The figure shows three views and two pictorial views of one solid part (mm, origin at its lowest corner). Answer the questions. A direction names the side the tool comes from. Round coordinates to 2 decimals unless told otherwise and drop trailing zeros. Order: outer loops, then holes, each group sorted by start corner. A loop starts at its lowest first (then second) coordinate and runs counter-clockwise, first axis right, second up. Notation, with made-up numbers: (-32, -8) -> (6, -8) arc R26 ccw to (6, 13) -> close; hole circle Ø7 at (-23.5, -24.75). An arc over 180 degrees is marked (long way). Return JSON: item names as keys, results as strings. Group by question number.
(1) Which of the six approach directions +Z, -Z, +X, -X, +Y, -Y give full straight-line access (tool end or side, diameter ignored) to the marked faces 1, 2, 3 and 4?
(2) Consider line 1 (Z direction, x = 5.5, y = 7); line 2 (X direction, y = 0.55, z = 4); line 3 (Z direction, x = 31, y = 7.25). Determine where each line is inside the solid, lowest interval first. Write a range as [from, to].
(3) The part is cut by section C-C (x = 9.5). Determine the outline of the cut face in (y, z), plus the area to 3 significant figures.
(4) Determine the mould class of the marked faces 5, 6 and 7 for opening direction X: +X half, -X half, draft (parallel to the pull), parting line (faces both ways), or undercut.
(5) Each of these flat-tipped pins is pushed along its axis until it touches: pin 1 (1 mm diameter, centred on x = 33, y = 6, fed in from -Z); pin 2 (0.6 mm diameter, centred on y = 1, z = 8, fed in from -X); pin 3 (4 mm diameter, centred on x = 28.5, z = 9, fed in from -Y). Where does it stop, or does it pass through?
(6) The part is cut by section D-D (z = 16.5). Determine the outline of the cut face in (x, y).
(7) The part is cut by section B-B (y = 5). Determine the outline of the cut face in (x, z), plus the area to 3 significant figures.
(8) The part is cut by section A-A (z = 34). Determine the outline of the cut face in (x, y), plus the area to 3 significant figures.
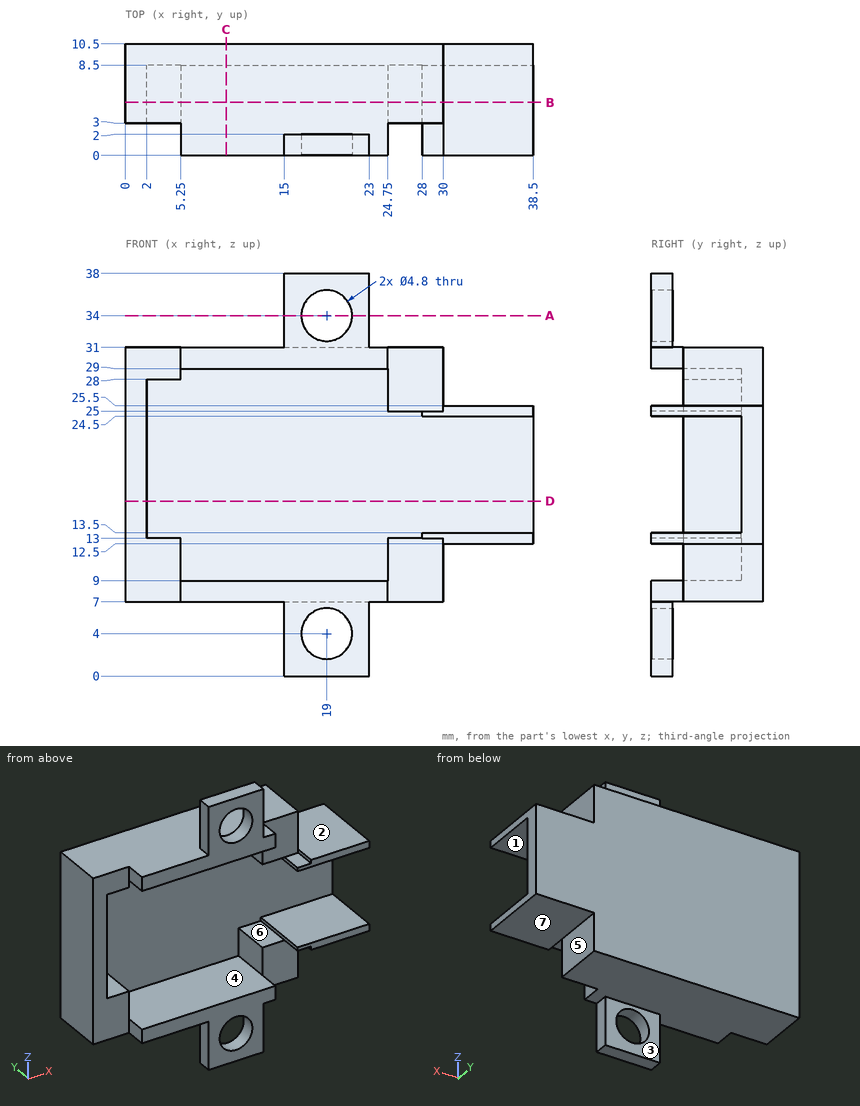
Answer below:
{
 "1": {"face 1": "+X, -Y", "face 2": "+Z, +X, +Y, -Y", "face 3": "-Z, +X, -X, +Y", "face 4": "-Y"},
 "2": {"line 1": "z = [7, 9], [29, 31]", "line 2": "x = [15, 16.6], [21.4, 23]", "line 3": "z = [12.5, 13.5], [24.5, 25.5]"},
 "3": {"outline": "(0, 7) -> (10.5, 7) -> (10.5, 31) -> (0, 31) -> (0, 29) -> (8.5, 29) -> (8.5, 9) -> (0, 9) -> close", "area": "82.0 mm²"},
 "4": {"face 5": "+X half", "face 6": "undercut", "face 7": "draft"},
 "5": {"pin 1": "stops at z = 12.5", "pin 2": "stops at x = 5.25", "pin 3": "stops at y = 3"},
 "6": {"outline": "(0, 3) -> (2, 3) -> (2, 8.5) -> (38.5, 8.5) -> (38.5, 10.5) -> (0, 10.5) -> close"},
 "7": {"outline": "(0, 7) -> (30, 7) -> (30, 12.5) -> (38.5, 12.5) -> (38.5, 13.5) -> (28, 13.5) -> (28, 13) -> (24.75, 13) -> (24.75, 9) -> (5.25, 9) -> (5.25, 13) -> (2, 13) -> (2, 28) -> (5.25, 28) -> (5.25, 29) -> (24.75, 29) -> (24.75, 25) -> (28, 25) -> (28, 24.5) -> (38.5, 24.5) -> (38.5, 25.5) -> (30, 25.5) -> (30, 31) -> (0, 31) -> close", "area": "237 mm²"},
 "8": {"outline": "(15, 0) -> (16.6, 0) -> (16.6, 2) -> (15, 2) -> close; (21.4, 0) -> (23, 0) -> (23, 2) -> (21.4, 2) -> close", "area": "6.40 mm²"}
}
